Autodesk Inventor part; units mm, degrees
ref_plane "Work Plane1" through (0, 0, 22.225) normal (-1, 0, 0) x (0, 0, 1)
sketch "Sketch1" plane through (0, 0, 0) normal (0, 1, 0) x (-1, 0, 0)
  line L0 (7.9375, 22.225) -> (-7.9375, 22.225)
  line L1 (-7.9375, 22.225) -> (-7.9375, -22.225)
  line L2 (-7.9375, -22.225) -> (7.9375, -22.225)
  line L3 (7.9375, -22.225) -> (7.9375, 22.225)
  line L4 (7.9375, 22.225) -> (-7.9375, -22.225) construction
  line L5 (-7.9375, 22.225) -> (7.9375, -22.225) construction
  point P0 (0, 0)
  point P1 (-50.8, 0)
  dimension "d0" = 15.875
  dimension "d1" = 44.45
extrude "Base" add sketch "Sketch1" along normal blind 4.7625
sketch "Sketch2" plane through (7.9375, 0, 22.225) normal (1, 0, 0) x (0, 0, -1)
  line L0 (0, 0) -> (0, 4.7625)
  line L1 (0, 4.7625) -> (10.2968, 32.9347)
  line L2 (0, 4.7625) -> (44.45, 4.7625)
  line L3 (34.1532, 32.9347) -> (44.45, 4.7625)
  line L4 (0, 0) -> (44.45, 0)
  arc A0 (34.1532, 32.9347) -> (10.2968, 32.9347) centre (22.225, 28.575) ccw
  line L5 (0, 0) -> (44.45, 0)
  line L6 (44.45, 0) -> (44.45, 4.7625)
  line L7 (0, 4.7625) -> (44.45, 4.7625)
  line L8 (0, 0) -> (0, 4.7625)
  point P0 (22.225, 0)
  point P1 (22.225, 41.275)
  dimension "d10" = 12.7
  dimension "d12" = 41.275
extrude "Vertical 1" add sketch "Sketch2" along normal blind 4.7625
sketch "Sketch5" plane through (-7.9375, 0, -22.225) normal (-1, 0, 0) x (0, 0, 1)
  line L0 (44.45, 4.7625) -> (44.45, 0)
  line L1 (44.45, 0) -> (0, 0)
  line L2 (0, 0) -> (0, 4.7625)
  line L3 (0, 4.7625) -> (10.2968, 32.9347)
  arc A0 (34.1532, 32.9347) -> (10.2968, 32.9347) centre (22.225, 28.575) ccw
  line L4 (34.1532, 32.9347) -> (44.45, 4.7625)
extrude "Vertical 2" add sketch "Sketch5" along normal blind 4.7625
sketch "Sketch6" plane through (12.7, 0, 22.225) normal (1, 0, 0) x (0, 0, -1)
  line L0 (22.225, 0) -> (22.225, 41.275) construction
  arc A0 (34.1532, 32.9347) -> (10.2968, 32.9347) centre (22.225, 28.575) ccw
  circle A1 centre (22.225, 31.75) radius 6.35
  dimension "d29" = 12.7
  dimension "d30" = 9.525
extrude "Extrusion8" cut sketch "Sketch6" against normal through all
fillet "Fillet2" radius 3.175 6 edges at (-12.7, 0, 0) (-12.7, 2.3813, -22.225) (12.7, 2.3813, -22.225) (12.7, 2.3813, 22.225) (12.7, 0, 0) (-12.7, 2.3813, 22.225)
chamfer "Chamfer2" distance 1.27 angle 45 2 edges at (-7.9375, 4.7625, 0) (7.9375, 4.7625, 0)
ref_plane "Work Plane2" through (0, 31.75, 0) normal (0, 1, 0) x (-1, 0, 0)
sketch "Sketch7" plane through (0, 4.7625, 0) normal (0, 1, 0) x (1, 0, 0)
  line L0 (0, 31.115) -> (0, -31.115) construction
  line L1 (17.78, 0) -> (-17.78, 0) construction
  point P0 (0, 0)
  point P1 (0, -15)
  point P2 (0, 15)
  dimension "d37" = 30
hole "Hole1" at (0, 4.7625, 15) at (0, 4.7625, -15) direction (0, -1, 0) diameter 6 end through all
ref_plane "Work Plane1" through (0, 0, 22.225) normal (-1, 0, 0) x (0, 0, 1)
equation "\"d43\" = Thickness"
equation "\"BendRadius\" = Thickness"
equation "\"BendReliefWidth\" = Thickness"
equation "\"BendReliefDepth\" = 0.5 * Thickness"
equation "\"CornerReliefSize\" = 4 * Thickness"
equation "\"MinimumRemnant\" = 2 * Thickness"
equation "\"TransitionRadius\" = BendRadius"
equation "\"JacobiRadiusSize\" = BendRadius"
equation "\"GapSize\" = Thickness"
properties part number "0.5 in Rod End Bracket (Rough)"
Work out the finished part from the listing and answer in its coordinate system (mm). A direction names the side the tool comes from. Give positions to 0.01 mm unless a question says otherwise; leave off trailing zeros. Write each loop counter-clockwise with the first axis right and the second up, starting at its lowest first coordinate (ties: lowest second). Pieces come first, ordered by that corner, then holes. Notation, with made-up numbers: (71, 10.25) - (86, 10.25) arc R19 cw to (86, 14.25) - close; hole circle Ø11 at (19.5, -9). An arc over 180 degrees is marked (long way). Use one line per item in the form item = value.
1. A cutting plane is placed at C-C (x = 0). Write down the section's boundary in (y, z) (1 decimal), and give its area (3 significant figures).
Filled in:
outline = (0, -22.2) - (4.8, -22.2) - (4.8, -18) - (0, -18) - close; (0, -12) - (4.8, -12) - (4.8, 12) - (0, 12) - close; (0, 18) - (4.8, 18) - (4.8, 22.2) - (0, 22.2) - close
area = 155 mm^2
2. Determine the mould class of faces 3 (the face through (-12.106, 5.136, 20.9)), 4 (the face through (-11.75, 0.91, -0.31)), 5 (the face through (0, 2, -18)) for opening direction Z: released by +Z, released by -Z, zero draft, split by the parting line, or undercut.
Filled in:
face_3 = released by +Z
face_4 = zero draft
face_5 = undercut
3. Consider L1, parallel to Z at x = 0, y = 1.8 (3 decimals); L2, parallel to X at y = 24.5, z = 11.5; L3, parallel to X at y = 4, z = -15. Determine where each line is inside the solid, lowest interval first.
Filled in:
L1 = -22.225 to -18, -12 to 12, 18 to 22.225
L2 = -12.7 to -7.94, 7.94 to 12.7
L3 = -12.7 to -3, 3 to 12.7
4. Each of these flat-tipped pins is pushed along its axis until it touches: pin 1 Ø7.5 at (y, z) = (31.75, 0) entering from -X; pin 2 Ø10 at (x, z) = (-9.5, -10) entering from +Y; pin 3 Ø6.5 at (x, z) = (0, 2) entering from +Y; pin 4 Ø10 at (x, y) = (6.5, 37) entering from -Z. Where does it stop, or does it pass through?
Filled in:
pin_1 = through
pin_2 = 40.25
pin_3 = 4.76
pin_4 = -12.19
5. A cutting plane is placed at B-B (y = 30). Write down the section's boundary in (x, z), and give its area (3 significant figures).
Filled in:
outline = (-12.7, -13) - (-7.94, -13) - (-7.94, -6.1) - (-12.7, -6.1) - close; (-12.7, 6.1) - (-7.94, 6.1) - (-7.94, 13) - (-12.7, 13) - close; (7.94, -13) - (12.7, -13) - (12.7, -6.1) - (7.94, -6.1) - close; (7.94, 6.1) - (12.7, 6.1) - (12.7, 13) - (7.94, 13) - close
area = 131 mm^2
6. A cutting plane is placed at A-A (z = 0). State how many separate pieces and enclosed holes the cut face has, and give its area (3 significant figures).
Filled in:
separate_pieces = 3
enclosed_holes = 0
area = 345 mm^2
7. For faces 1 (the face through (-7.311, 5.406, 0.311)), 2 (the face through (0, 2, 12)), determine the directions among +Z, -Z, +X, -X, +Y, -Y from which every point of the face is accessible in a straight line to the end or side of a thin tool.
Filled in:
face_1 = +Z, -Z, +Y
face_2 = +Y, -Y
